from build123d import *

# Parameters (mm, degrees)
EXTRUDE_1_DEPTH               = 2
HOLE_WIZARD_M2_51_AT_2_COUNT  = 2
HOLE_WIZARD_M2_51_AT_2_PITCH  = 16.931296872
HOLE_WIZARD_M2_51_AT_3_COUNT  = 2
HOLE_WIZARD_M2_51_AT_3_PITCH  = 35.210867013
HOLE_WIZARD_M2_51_AT_4_COUNT  = 2
HOLE_WIZARD_M2_51_AT_4_PITCH  = 59.977461264
HOLE_WIZARD_M2_51_AT_5_COUNT  = 2
HOLE_WIZARD_M2_51_AT_5_PITCH  = 77.079878905
HOLE_WIZARD_M2_51_AT_6_COUNT  = 2
HOLE_WIZARD_M2_51_AT_6_PITCH  = 88.813353391
HOLE_WIZARD_M2_51_AT_7_COUNT  = 2
HOLE_WIZARD_M2_51_AT_7_PITCH  = 85.825277806
HOLE_WIZARD_M2_51_AT_8_COUNT  = 2
HOLE_WIZARD_M2_51_AT_8_PITCH  = 68.275845665
HOLE_WIZARD_M2_51_AT_9_COUNT  = 2
HOLE_WIZARD_M2_51_AT_9_PITCH  = 40.65296425
HOLE_WIZARD_M2_51_AT_10_COUNT = 2
HOLE_WIZARD_M2_51_AT_10_PITCH = 30.544658358
HOLE_WIZARD_M2_51_AT_11_COUNT = 2
HOLE_WIZARD_M2_51_AT_11_PITCH = 58.937345854
HOLE_WIZARD_M2_51_AT_12_COUNT = 2
HOLE_WIZARD_M2_51_AT_12_PITCH = 111.179377124
HOLE_WIZARD_M2_51_AT_13_COUNT = 2
HOLE_WIZARD_M2_51_AT_13_PITCH = 99.231085308
CUT_EXTRUDE_1_DEPTH           = 143.22856359
CUT_EXTRUDE_1_DEPTH_BACK      = 143.22856359


with BuildPart() as part:
    # Outline → Бобышка-Вытянуть1 (new body)
    with BuildSketch(Plane.XY):
        with BuildLine():
            Line((12.02500062, 78.2), (0, 78.2))
            ThreePointArc((0, 78.2), (-9.333809512, 74.333809512), (-13.2, 65))
            Line((-13.2, 65), (-13.2, 0))
            ThreePointArc((-13.2, 0), (-9.333809512, -9.333809512), (0, -13.2))
            Line((0, -13.2), (105, -13.2))
            ThreePointArc((105, -13.2), (114.333809512, -9.333809512), (118.2, 0))
            Line((118.2, 0), (118.2, 65))
            ThreePointArc((118.2, 65), (114.333809512, 74.333809512), (105, 78.2))
            Line((105, 78.2), (12.02500062, 78.2))
        make_face()
    extrude(amount=EXTRUDE_1_DEPTH)

    # Эскиз8 → Отверстие с зазором M2.51 (revolve, cut)
    with BuildSketch(Plane(origin=(14.552676738, 48.9918182, 2), x_dir=(0, -1, 0), z_dir=(1, 0, 0))):
        Polygon((0, 0), (0, 2), (1.45, 2), (1.45, 1.3), (2.75, 0), align=None)
    hole_wizard_m2_51 = revolve(axis=Axis((14.552676738, 48.9918182, 8.35), (0, 0, -1)), mode=Mode.SUBTRACT)

    # Отверстие с зазором M2.51 at 2: Отверстие с зазором M2.51 ×2
    with Locations(*[Vector(-0.17005574614353655, -0.9854344438893767, 0) * (i * HOLE_WIZARD_M2_51_AT_2_PITCH) for i in range(1, HOLE_WIZARD_M2_51_AT_2_COUNT)]):
        add(hole_wizard_m2_51, mode=Mode.SUBTRACT)

    # Отверстие с зазором M2.51 at 3: Отверстие с зазором M2.51 ×2
    with Locations(*[Vector(0.6774960962058836, -0.7355263690893673, 0) * (i * HOLE_WIZARD_M2_51_AT_3_PITCH) for i in range(1, HOLE_WIZARD_M2_51_AT_3_COUNT)]):
        add(hole_wizard_m2_51, mode=Mode.SUBTRACT)

    # Отверстие с зазором M2.51 at 4: Отверстие с зазором M2.51 ×2
    with Locations(*[Vector(0.8296904036666649, -0.5582238207596005, 0) * (i * HOLE_WIZARD_M2_51_AT_4_PITCH) for i in range(1, HOLE_WIZARD_M2_51_AT_4_COUNT)]):
        add(hole_wizard_m2_51, mode=Mode.SUBTRACT)

    # Отверстие с зазором M2.51 at 5: Отверстие с зазором M2.51 ×2
    with Locations(*[Vector(0.8255988861757253, -0.5642574582098157, 0) * (i * HOLE_WIZARD_M2_51_AT_5_PITCH) for i in range(1, HOLE_WIZARD_M2_51_AT_5_COUNT)]):
        add(hole_wizard_m2_51, mode=Mode.SUBTRACT)

    # Отверстие с зазором M2.51 at 6: Отверстие с зазором M2.51 ×2
    with Locations(*[Vector(0.9202423986359286, -0.3913488568436004, 0) * (i * HOLE_WIZARD_M2_51_AT_6_PITCH) for i in range(1, HOLE_WIZARD_M2_51_AT_6_COUNT)]):
        add(hole_wizard_m2_51, mode=Mode.SUBTRACT)

    # Отверстие с зазором M2.51 at 7: Отверстие с зазором M2.51 ×2
    with Locations(*[Vector(0.9746234007113833, -0.22385090302649743, 0) * (i * HOLE_WIZARD_M2_51_AT_7_PITCH) for i in range(1, HOLE_WIZARD_M2_51_AT_7_COUNT)]):
        add(hole_wizard_m2_51, mode=Mode.SUBTRACT)

    # Отверстие с зазором M2.51 at 8: Отверстие с зазором M2.51 ×2
    with Locations(*[Vector(0.9740559678514582, -0.22630725019972095, 0) * (i * HOLE_WIZARD_M2_51_AT_8_PITCH) for i in range(1, HOLE_WIZARD_M2_51_AT_8_COUNT)]):
        add(hole_wizard_m2_51, mode=Mode.SUBTRACT)

    # Отверстие с зазором M2.51 at 9: Отверстие с зазором M2.51 ×2
    with Locations(*[Vector(0.9447489174324829, -0.327794879475186, 0) * (i * HOLE_WIZARD_M2_51_AT_9_PITCH) for i in range(1, HOLE_WIZARD_M2_51_AT_9_COUNT)]):
        add(hole_wizard_m2_51, mode=Mode.SUBTRACT)

    # Отверстие с зазором M2.51 at 10: Отверстие с зазором M2.51 ×2
    with Locations(*[Vector(-0.6814719875063323, 0.73184419806689, 0) * (i * HOLE_WIZARD_M2_51_AT_10_PITCH) for i in range(1, HOLE_WIZARD_M2_51_AT_10_COUNT)]):
        add(hole_wizard_m2_51, mode=Mode.SUBTRACT)

    # Отверстие с зазором M2.51 at 11: Отверстие с зазором M2.51 ×2
    with Locations(*[Vector(-0.35317723825652403, -0.9355564324921798, 0) * (i * HOLE_WIZARD_M2_51_AT_11_PITCH) for i in range(1, HOLE_WIZARD_M2_51_AT_11_COUNT)]):
        add(hole_wizard_m2_51, mode=Mode.SUBTRACT)

    # Отверстие с зазором M2.51 at 12: Отверстие с зазором M2.51 ×2
    with Locations(*[Vector(0.8683521022085285, -0.49594820958445784, 0) * (i * HOLE_WIZARD_M2_51_AT_12_PITCH) for i in range(1, HOLE_WIZARD_M2_51_AT_12_COUNT)]):
        add(hole_wizard_m2_51, mode=Mode.SUBTRACT)

    # Отверстие с зазором M2.51 at 13: Отверстие с зазором M2.51 ×2
    with Locations(*[Vector(0.9742960388993211, 0.2252714553268849, 0) * (i * HOLE_WIZARD_M2_51_AT_13_PITCH) for i in range(1, HOLE_WIZARD_M2_51_AT_13_COUNT)]):
        add(hole_wizard_m2_51, mode=Mode.SUBTRACT)

    # Эскиз10 → Вырез-Вытянуть1 (cut, two sides: drawn at the far end of the back side and taken through both)
    with BuildSketch(Plane.XY.offset(-9.9366788).offset(-CUT_EXTRUDE_1_DEPTH_BACK)):
        with BuildLine():
            Line((80.689492233, 74.5), (97.346654465, 74.5))
            ThreePointArc((97.346654465, 74.5), (98.760868027, 73.914213562), (99.346654465, 72.5))
            Line((99.346654465, 72.5), (99.346654465, 60.572687633))
            ThreePointArc((99.346654465, 60.572687633), (98.760868027, 59.158474071), (97.346654465, 58.572687633))
            Line((97.346654465, 58.572687633), (80.689492233, 58.572687633))
            ThreePointArc((80.689492233, 58.572687633), (79.275278671, 59.158474071), (78.689492233, 60.572687633))
            Line((78.689492233, 60.572687633), (78.689492233, 72.5))
            ThreePointArc((78.689492233, 72.5), (79.275278671, 73.914213562), (80.689492233, 74.5))
        make_face()
    extrude(amount=CUT_EXTRUDE_1_DEPTH + CUT_EXTRUDE_1_DEPTH_BACK, mode=Mode.SUBTRACT)


solid = part.part
Can you work these out from the model? Positions are in its coordinate system, mm. Coordinates: 2 decimals unless noted, no trailing zeros. Write each loop counter-clockwise with the first axis right and the second up, starting at its lowest first coordinate (ties: lowest second). Pieces come first, ordered by that corner, then holes. Notation, with made-up numbers: (-39.75, -35) -> (7.25, -35) arc R34 ccw to (7.25, -1) -> close; hole circle Ø2 at (8.5, 59). An arc over 180 degrees is marked (long way). Write each question's results on one line, items separated by ' | '. Start each with the question number.
Item 1: Thinking about a two-plate mould opening in Y: for faces 1 (the cylindrical face through (99.616, 30.094, 0.355)), 2 (the flat face through (52, 33, 0)), 3 (the cylindrical face through (114.231, -9.436, 0.986)), which applies, released by +Y, released by -Y, zero draft, split by the parting line, or undercut?
Item 2: I'm going to push flat-ended pins straight in: P1, Ø4.5, axis at x = 14.55, y = 48.99, coming from the -Z side; P2, Ø2.5, axis at x = 38.41, y = 23.09, coming from the -Z side; P3, Ø4.5, axis at x = 98.2, y = 29.78, coming from the +Z side. Where does each tip first touch, or does it pass through?
Item 3: If we section it at B-B, the plane z = 1.3: Count the separate pieces of the cut face and the enclosed holes in it, and give its area (3 significant figures).
Item 4: If we section it at A-A, the plane y = 62: Write out the boundary of the cut face in (x, z), and give its area (3 significant figures).
Item 5: Please list where these lines run through material, in increasing order: probe 1 along X at (y, z) = (64, 0.35); probe 2 along Y at (x, z) = (95, 0.85); probe 3 along Y at (x, z) = (98, 0.3).
Answer block:
1) face 1: undercut | face 2: zero draft | face 3: released by -Y
2) P1: z = 0 | P2: through | P3: z = 1.5
3) separate pieces: 1 | enclosed holes: 14 | area: 11,400 mm²
4) outline: (-13.2, 0) -> (78.69, 0) -> (78.69, 2) -> (-13.2, 2) -> close; (99.35, 0) -> (118.2, 0) -> (118.2, 2) -> (99.35, 2) -> close | area: 221 mm²
5) probe 1: -13.2 to 78.69, 99.35 to 118.2 | probe 2: -13.2 to 13.28, 15.19 to 58.57, 74.5 to 78.2 | probe 3: -13.2 to 28.34, 31.22 to 58.68, 74.39 to 78.2
